from build123d import *

# Parameters (mm, degrees)
SKETCH2_R          = 7.5
CUT_EXTRUDE2_DEPTH = 29.7


with BuildPart() as part:
    # Sketch1 → Revolve1 (revolve)
    with BuildSketch(Plane(origin=(0, 0, 0), x_dir=(0, 0, -1), z_dir=(1, 0, 0))):
        Polygon((-6.45, 6), (0, 6), (0, 0), (3.075, 0), (3.075, -2.009350098), (8.125, -2.009350098), (8.125, 0), (14.125, 0), (14.125, -2.009350098), (19.175, -2.009350098), (19.175, 0), (22.25, 0), (22.25, -7.6), (0, -7.6), (0, -51), (-6.45, -51), align=None)
    revolve(axis=Axis((0, -51, 6.45), (0, 0, -1)))

    # Sketch2 → Cut-Extrude2 (cut, through all)
    with BuildSketch(Plane.XY.offset(6.45)):
        with Locations((18, -51)):
            Circle(SKETCH2_R)
        with Locations((-18, -51)):
            Circle(SKETCH2_R)
    extrude(amount=-CUT_EXTRUDE2_DEPTH, mode=Mode.SUBTRACT)


solid = part.part
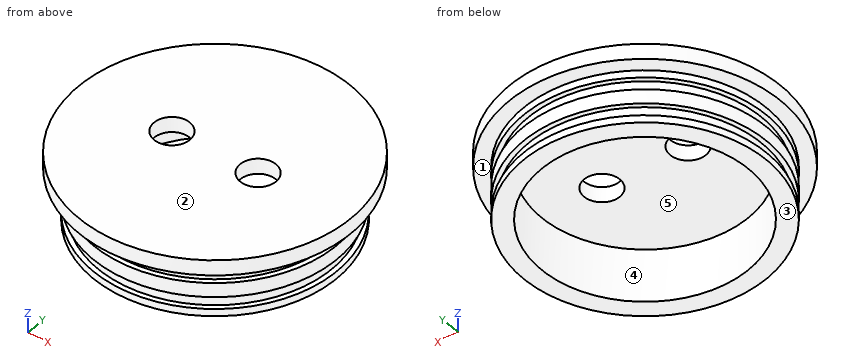
Read the model definition and answer for the solid it produces. Units are mm, in the model's axes. Face numbers are marked on the shaded views. A direction names the side the tool comes from. Round coordinates to 2 decimals unless told otherwise and drop trailing zeros. Write each loop counter-clockwise with the first axis right and the second up, starting at its lowest first coordinate (ties: lowest second). Pieces come first, ordered by that corner, then holes. Notation, with made-up numbers: (87, -20) - (133, -20) arc R17 cw to (133, -6) - close; hole circle Ø7 at (89, 71.25). An arc over 180 degrees is marked (long way). One line per question, with ' | ' between items. Start each with the question number.
1. For a pull along X with two mould halves and no side action, classify the marked faces 3, 4 and 5 as +X half, -X half, draft (parallel to the pull), parting line (faces both ways), or undercut.
2. Section C-C (x = 0) is taken. Determine the outline of the cut face in (y, z) (3 decimals).
3. Section B-B (y = -51) is taken. Give the number of separate pieces and of enclosed holes in the cut face, and give its area (3 significant figures).
4. For the marked faces 1 and 2, determine the directions among +Z, -Z, +X, -X, +Y, -Y from which every point of the face is accessible in a straight line to the end or side of a thin tool.
5. Each of these flat-tipped pins is pushed along its axis until it touches: pin 1 (1.5 mm diameter, centred on y = -92.5, z = -15, fed in from -X); pin 2 (1.5 mm diameter, centred on y = -93, z = -19, fed in from +X); pin 3 (12 mm diameter, centred on x = 44.5, z = 1.5, fed in from -Y); pin 4 (13.5 mm diameter, centred on x = -18, y = -51, fed in from +Z). Where does it stop, or does it pass through?
6. Section D-D (y = -27) is taken. Determine the outline of the cut face in (x, z) (3 decimals), and give its area (3 significant figures).
7. Find the intervals of material crossed by probe 1 along X at (y, z) = (-51, -9.75); probe 2 along X at (y, z) = (-52, -8); probe 3 along Z at (x, y) = (18, -89), in increasing order. Write a range as [from, to].
Filled in:
1) face 3: draft | face 4: undercut | face 5: undercut
2) outline: (-108, 0) - (-102, 0) - (-102, -3.075) - (-99.991, -3.075) - (-99.991, -8.125) - (-102, -8.125) - (-102, -14.125) - (-99.991, -14.125) - (-99.991, -19.175) - (-102, -19.175) - (-102, -22.25) - (-94.4, -22.25) - (-94.4, 0) - (-7.6, 0) - (-7.6, -22.25) - (0, -22.25) - (0, -19.175) - (-2.009, -19.175) - (-2.009, -14.125) - (0, -14.125) - (0, -8.125) - (-2.009, -8.125) - (-2.009, -3.075) - (0, -3.075) - (0, 0) - (6, 0) - (6, 6.45) - (-108, 6.45) - close
3) separate pieces: 3 | enclosed holes: 0 | area: 839 mm²
4) face 1: -Z | face 2: +Z, +X, -X, +Y, -Y
5) pin 1: x = -27.19 | pin 2: x = 29.96 | pin 3: y = -93.03 | pin 4: through
6) outline: (-51.701, 0) - (-45, 0) - (-45, -3.075) - (-42.709, -3.075) - (-42.709, -8.125) - (-45, -8.125) - (-45, -14.125) - (-42.709, -14.125) - (-42.709, -19.175) - (-45, -19.175) - (-45, -22.25) - (-36.16, -22.25) - (-36.16, 0) - (36.16, 0) - (36.16, -22.25) - (45, -22.25) - (45, -19.175) - (42.709, -19.175) - (42.709, -14.125) - (45, -14.125) - (45, -8.125) - (42.709, -8.125) - (42.709, -3.075) - (45, -3.075) - (45, 0) - (51.701, 0) - (51.701, 6.45) - (-51.701, 6.45) - close | area: 1,010 mm²
7) probe 1: [-51, -43.4], [43.4, 51] | probe 2: [-48.98, -43.39], [43.39, 48.98] | probe 3: [0, 6.45]
